```python
from build123d import *

# Parameters (mm, degrees)
EXTRUDE_TOP_BLOCK_DEPTH             = 75
CUT_EXTRUDE_BOLT_PATTERN_DEPTH      = 108.574034239
CUT_EXTRUDE_BOLT_PATTERN_DEPTH_BACK = 108.574034239
SKETCH2_R                           = 2.75
EXTRUDE_START                       = -16
EXTRUDE_ADDITION_MATERIAL_DEPTH     = 59
CUT_EXTRUDE_SHAFT_PATHWAY_REACH     = 99.296
SKETCH7_R                           = 2
CUT_EXTRUDE1_DEPTH                  = 25
SKETCH8_R                           = 4.5
CUT_EXTRUDE2_DEPTH                  = 6


with BuildPart() as part:
    # Sketch1 → Extrude Top Block (new body)
    with BuildSketch(Plane(origin=(0, 0, 0), x_dir=(1, 0, 0), z_dir=(0, 0.13052619222003847, 0.9914448613738122))):
        with BuildLine():
            Line((62.5, 0.75), (62.5, 37.5))
            Line((62.5, 37.5), (-62.5, 37.5))
            Line((-62.5, 37.5), (-62.5, 0.75))
            Line((-62.5, 0.75), (-26.489384666, 0.75))
            ThreePointArc((-26.489384666, 0.75), (0, 26.5), (26.489384666, 0.75))
            Line((26.489384666, 0.75), (62.5, 0.75))
        make_face()
    extrude(amount=-EXTRUDE_TOP_BLOCK_DEPTH)

    # Sketch2 → Cut-Extrude Bolt Pattern (cut, two sides: drawn at the far end of the back side and taken through both)
    with BuildSketch(Plane(origin=(0, 37.179182302, -4.894732208), x_dir=(1, 0, 0), z_dir=(0, 0.9914448613738122, -0.13052619222003847)).offset(-CUT_EXTRUDE_BOLT_PATTERN_DEPTH_BACK)):
        with Locations(Location((-47.5, 15, 0), (0, 0, 270))):
            Circle(SKETCH2_R)
        with Locations(Location((-47.5, 60, 0), (0, 0, 270))):
            Circle(SKETCH2_R)
        with Locations(Location((47.5, 15, 0), (0, 0, 270))):
            Circle(SKETCH2_R)
        with Locations(Location((47.5, 60, 0), (0, 0, 270))):
            Circle(SKETCH2_R)
    extrude(amount=CUT_EXTRUDE_BOLT_PATTERN_DEPTH + CUT_EXTRUDE_BOLT_PATTERN_DEPTH_BACK, mode=Mode.SUBTRACT)

    # Sketch4 → Extrude Addition Material (add)
    with BuildSketch(Plane(origin=(0, 0, 0), x_dir=(1, 0, 0), z_dir=(0, 0.13052619222003847, 0.9914448613738122)).offset(EXTRUDE_START)):
        with BuildLine():
            Line((-26.489384666, 0.75), (26.489384666, 0.75))
            ThreePointArc((26.489384666, 0.75), (0, 26.5), (-26.489384666, 0.75))
        make_face()
    extrude(amount=-EXTRUDE_ADDITION_MATERIAL_DEPTH)

    # Sketch3 → Cut-Extrude Seat for Linear Bearing (revolve, cut)
    with BuildSketch(Plane(origin=(0, 0, 0), x_dir=(0, 0, -1), z_dir=(1, 0, 0))):
        Polygon((41.497659566, 1.092817718), (61.326556793, -1.517706126), (60.478136544, -7.962097725), (40.649239316, -5.351573881), align=None)
    revolve(axis=Axis((0, 0, 0), (0, -0.1305261922200383, -0.9914448613738122)), mode=Mode.SUBTRACT)

    # Cut-Extrude Shaft Pathway: up to this face of the body (flat: up to its plane)
    cut_extrude_shaft_pathway_end = Plane(part.part.faces().sort_by_distance((0, 9.171918557, -76.854678029))[0])
    # Sketch6 → Cut-Extrude Shaft Pathway (cut, up to the picked face)
    with BuildSketch(Plane(origin=(0, -2.088419076, -15.863117782), x_dir=(1, 0, 0), z_dir=(0, 0.13052619222003847, 0.9914448613738122)), mode=Mode.PRIVATE) as cut_extrude_shaft_pathway_sk1:
        with BuildLine():
            Line((-4.943429983, 0.75), (4.943429983, 0.75))
            ThreePointArc((4.943429983, 0.75), (0, 5), (-4.943429983, 0.75))
        make_face()
    cut_extrude_shaft_pathway_tool1 = split(extrude(cut_extrude_shaft_pathway_sk1.sketch, amount=-CUT_EXTRUDE_SHAFT_PATHWAY_REACH, mode=Mode.PRIVATE), bisect_by=cut_extrude_shaft_pathway_end, keep=Keep.BOTH, mode=Mode.PRIVATE)
    add(cut_extrude_shaft_pathway_tool1.solids().sort_by(Axis((0, 0.422663, -16.193708), (0, -0.13052619222003847, -0.9914448613738122)))[0], mode=Mode.SUBTRACT)

    # Sketch7 → Cut-Extrude1 (cut)
    with BuildSketch(Plane(origin=(0, -9.789464417, -74.358364603), x_dir=(-1, 0, 0), z_dir=(0, -0.13052619222003847, -0.9914448613738122))):
        with Locations(Location((-20, 20, 0), (0, 0, 90))):
            Circle(SKETCH7_R)
        with Locations(Location((20, 20, 0), (0, 0, 90))):
            Circle(SKETCH7_R)
    extrude(amount=-CUT_EXTRUDE1_DEPTH, mode=Mode.SUBTRACT)

    # Sketch8 → Cut-Extrude2 (cut)
    with BuildSketch(Plane(origin=(0, 37.179182302, -4.894732208), x_dir=(1, 0, 0), z_dir=(0, 0.9914448613738122, -0.13052619222003847))):
        with Locations(Location((47.5, 15, 0), (0, 0, 270))):
            Circle(SKETCH8_R)
        with Locations(Location((47.5, 60, 0), (0, 0, 270))):
            Circle(SKETCH8_R)
        with Locations(Location((-47.5, 15, 0), (0, 0, 270))):
            Circle(SKETCH8_R)
        with Locations(Location((-47.5, 60, 0), (0, 0, 270))):
            Circle(SKETCH8_R)
    extrude(amount=-CUT_EXTRUDE2_DEPTH, mode=Mode.SUBTRACT)


solid = part.part
```
Input: part model. Units: mm. Frame: model coordinates. A direction names the side the tool comes from. Give positions to 0.01 mm unless a question says otherwise; leave off trailing zeros. Loops run counter-clockwise (first coordinate to the right, second up) from the corner with the lowest first, then second, coordinate; pieces in that order, holes last. Notation, with made-up numbers: M 2,72.25 L 35,72.25 A27 ccw 35,97.25 Z; hole C -21.75,-5.5 d6. An arc over 180 degrees is marked long. Answer as CSV lines item,"result". Start each with the question number.
1. Pull-direction query (Z, two-part tool) for faces 1 (the face through (-0.875, 27.313, -3.596)), 2 (the face through (-51.893, 32.161, -20.347)), 3 (the face through (-62.5, 14, -39)), 4 (the face through (0.875, 32.353, -41.553)); classes: released by +Z, released by -Z, zero draft, split by the parting line, or undercut.
2. Section B-B on y = 20. State how many separate pieces and enclosed holes the cut face has, plus the area to 3 significant figures.
3. Reachability of faces 5 (the face through (-0.37, 8.76, -17.29)), 6 (the face through (0.099, -3.907, -67.974)), 7 (the face through (-47.44, 23.78, -60.69)) from +Z, -Z, +X, -X, +Y, -Y: full face, straight path, thin tool, end or side. Return the list, or none.
4. Line query: L1, parallel to X at y = -5, z = -61; L2, parallel to Z at x = 48.5, y = 12.5; L3, parallel to Z at x = -47, y = 22. Output: solid intervals per line, ascending.
5. Pin query (flat end, axial travel): P1, Ø6, axis at x = -24, y = -4.5, coming from the -Z side; P2, Ø4, axis at x = 13.5, z = -28.5, coming from the -Y side; P3, Ø1.5, axis at x = 16, z = -54, coming from the +Y side. Return the tip coordinate at first contact, or that it passes through.
6. Section A-A on x = 10.5. Return loops of the section in (y, z).
Computed values:
1,face 1,"released by +Z"
1,face 2,"undercut"
1,face 3,"zero draft"
1,face 4,"released by -Z"
2,separate pieces,"1"
2,enclosed holes,"4"
2,area,"8,850 mm²"
3,face 5,"+Z"
3,face 6,"+Z, -Y"
3,face 7,"none"
4,L1,"x = -62.5 to -50.01, -44.99 to -4, 4 to 44.99, 50.01 to 62.5"
4,L2,"z = -77.29 to -64.75, -59.58 to -19.36, -14.19 to -1.65"
4,L3,"z = -78.54 to -66.14, -60.69 to -20.75, -15.3 to -2.9"
5,P1,"stops at z = -75.45"
5,P2,"stops at y = -3.26"
5,P3,"stops at y = 30.81"
6,outline,"M -9.05,-74.46 L 27.39,-79.25 L 37.18,-4.89 L 24.12,-3.18 L 22.03,-19.04 L -1.34,-15.96 Z"
